The figure shows three views and two pictorial views of one solid part (mm, origin at its lowest corner). Answer the questions. A direction names the side the tool comes from. Round coordinates to 2 decimals unless told otherwise and drop trailing zeros. Write each loop counter-clockwise with the first axis right and the second up, starting at its lowest first coordinate (ties: lowest second). Pieces come first, ordered by that corner, then holes.
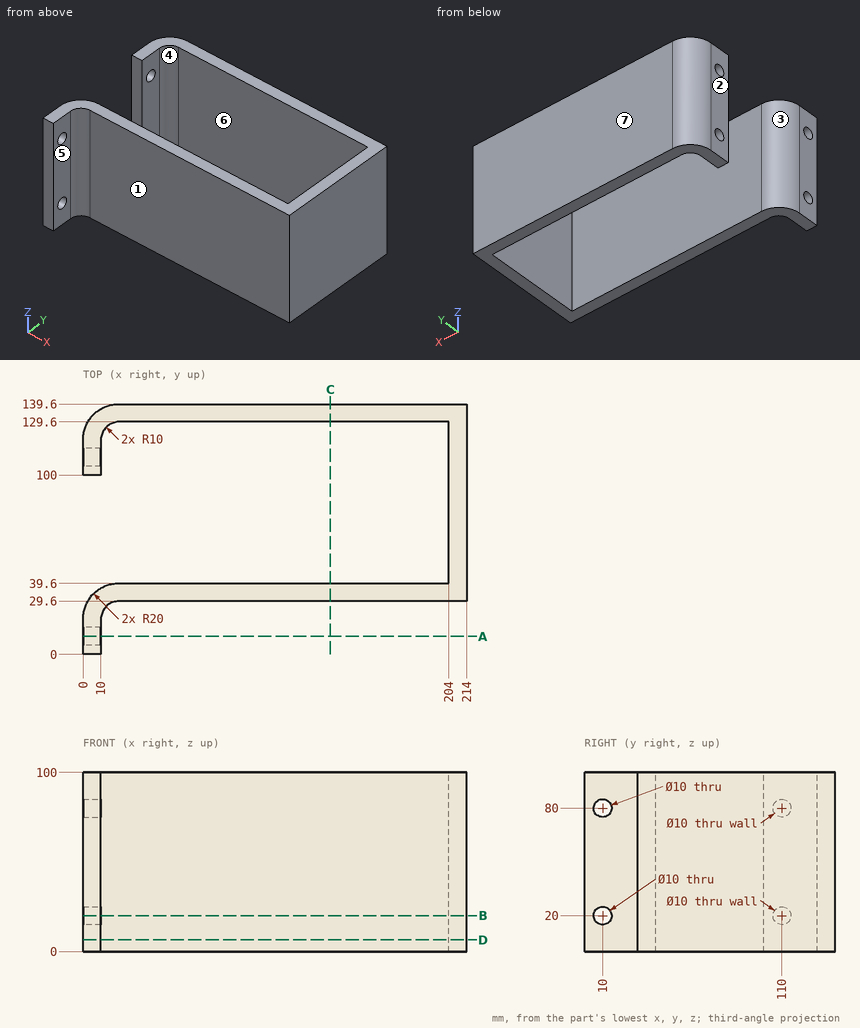
Q1. Section D-D (z = 6.5) is taken. Determine the outline of the cut face in (x, y), then the cut area to 3 significant figures.
Verdict:
outline: (0, 0) - (10, 0) - (10, 19.6) arc R10 cw to (20, 29.6) - (214, 29.6) - (214, 139.6) - (20, 139.6) arc R20 ccw to (0, 119.6) - (0, 100) - (10, 100) - (10, 119.6) arc R10 cw to (20, 129.6) - (204, 129.6) - (204, 39.6) - (20, 39.6) arc R20 ccw to (0, 19.6) - close
area: 5,640 mm2
Q2. Section B-B (z = 20) is taken. Determine the outline of the cut face in (x, y).
Verdict:
outline: (0, 0) - (10, 0) - (10, 5) - (0, 5) - close; (0, 15) - (10, 15) - (10, 19.6) arc R10 cw to (20, 29.6) - (214, 29.6) - (214, 139.6) - (20, 139.6) arc R20 ccw to (0, 119.6) - (0, 115) - (10, 115) - (10, 119.6) arc R10 cw to (20, 129.6) - (204, 129.6) - (204, 39.6) - (20, 39.6) arc R20 ccw to (0, 19.6) - close; (0, 100) - (10, 100) - (10, 105) - (0, 105) - close
Q3. Which of the six approach directions +Z, -Z, +X, -X, +Y, -Y give full straight-line access (tool end or side, diameter ignored) to the marked faces 1, 2, 3 and 4?
Verdict:
face 1: +Z, -Z, +X, -Y
face 2: +Z, -Z, -X, +Y, -Y
face 3: +Z, -Z, -X
face 4: +Z, -Z
Q4. Straight lines are drawn through the part: probe 1 along X at (y, z) = (107, 5.5); probe 2 along Y at (x, z) = (2.75, 80); probe 3 along Y at (x, z) = (28, 92). For each, find the intervals that lie inside material, in ascending order.
Verdict:
probe 1: x = 0 to 10, 204 to 214
probe 2: y = 0 to 5, 15 to 29.72, 100 to 105, 115 to 129.72
probe 3: y = 29.6 to 39.6, 129.6 to 139.6
Q5. Flat-ended cylindrical pins translate along their axes: pin 1 Ø16 at (y, z) = (110, 80) entering from -X; pin 2 Ø5 at (x, z) = (116.5, 74) entering from -Y; pin 3 Ø9 at (y, z) = (10, 20) entering from -X; pin 4 Ø21.5 at (y, z) = (11.5, 68.5) entering from +X. Find the tip coordinate at first contact, or state that the pin passes through.
Verdict:
pin 1: stops at x = 0
pin 2: stops at y = 29.6
pin 3: passes through
pin 4: stops at x = 10.36
Q6. Determine the mould class of the marked faces 5, 6 and 7 for opening direction Y: pulls with the +Y half, pulls with the -Y half, needs draft (parallel to the pull), parting line crosses it, or undercut.
Verdict:
face 5: needs draft
face 6: undercut
face 7: pulls with the +Y half
Q7. Section A-A (y = 10) is taken. Determine the outline of the cut face in (x, z), then the cut area to 3 significant figures.
Verdict:
outline: (0, 0) - (10, 0) - (10, 15) - (0, 15) - close; (0, 25) - (10, 25) - (10, 75) - (0, 75) - close; (0, 85) - (10, 85) - (10, 100) - (0, 100) - close
area: 800 mm2
Q8. Section C-C (x = 138) is taken. Determine the outline of the cut face in (y, z).
Verdict:
outline: (29.6, 0) - (39.6, 0) - (39.6, 100) - (29.6, 100) - close; (129.6, 0) - (139.6, 0) - (139.6, 100) - (129.6, 100) - close
